from build123d import *

# Parameters (mm, degrees)
BOX001_W          = 17
BOX001_H          = 14.6
BOX001_DEPTH      = 16.5
CYLINDER005_R     = 2.1
CYLINDER005_DEPTH = 2
CYLINDER004_R     = 2.1
CYLINDER004_DEPTH = 2
CYLINDER007_R     = 3.5
CYLINDER007_DEPTH = 0.75
BOX_W             = 7
BOX_H             = 35
BOX_DEPTH         = 0.75
CYLINDER006_R     = 3.5
CYLINDER006_DEPTH = 0.75
CYLINDER001_R     = 4.5
CYLINDER001_DEPTH = 1.5
CYLINDER_R        = 14
CYLINDER_DEPTH    = 19
BOX003_W          = 1
BOX003_H          = 5
BOX003_DEPTH      = 6
BOX002_W          = 1
BOX002_H          = 5
BOX002_DEPTH      = 6
CYLINDER003_R     = 2.5
CYLINDER003_DEPTH = 8.5


with BuildPart() as cube001:
    # Box001 → Box001 (new body)
    with BuildSketch(Plane(origin=(0, -7.3, 2.5), x_dir=(1, 0, 0), z_dir=(0, 0, 1))):
        with Locations((8.5, 7.3)):
            Rectangle(BOX001_W, BOX001_H)
    extrude(amount=BOX001_DEPTH)


with BuildPart() as cylinder005:
    # Cylinder005 → Cylinder005 (new body)
    with BuildSketch(Plane(origin=(0, 17.5, 18), x_dir=(1, 0, 0), z_dir=(0, 0, 1))):
        Circle(CYLINDER005_R)
    extrude(amount=CYLINDER005_DEPTH)


with BuildPart() as cylinder004:
    # Cylinder004 → Cylinder004 (new body)
    with BuildSketch(Plane(origin=(0, -17.5, 18), x_dir=(1, 0, 0), z_dir=(0, 0, 1))):
        Circle(CYLINDER004_R)
    extrude(amount=CYLINDER004_DEPTH)


with BuildPart() as cylinder007:
    # Cylinder007 → Cylinder007 (new body)
    with BuildSketch(Plane(origin=(0, 17.5, 18), x_dir=(1, 0, 0), z_dir=(0, 0, 1))):
        Circle(CYLINDER007_R)
    extrude(amount=CYLINDER007_DEPTH)


with BuildPart() as cube:
    # Box → Box (new body)
    with BuildSketch(Plane(origin=(-3.5, -17.5, 18), x_dir=(1, 0, 0), z_dir=(0, 0, 1))):
        with Locations((3.5, 17.5)):
            Rectangle(BOX_W, BOX_H)
    extrude(amount=BOX_DEPTH)


with BuildPart() as cut001:
    # Cylinder006 → Cylinder006 (new body)
    with BuildSketch(Plane(origin=(0, -17.5, 18), x_dir=(1, 0, 0), z_dir=(0, 0, 1))):
        Circle(CYLINDER006_R)
    extrude(amount=CYLINDER006_DEPTH)

    # Fusion: union Cylinder007, Cube
    add(cylinder007.part)
    add(cube.part)


with BuildPart() as cut001_1:
    # Fusion placement: moved
    add(cut001.part.moved(Location((0, 0, 0.25))))

    # Cut: cut Cylinder004
    add(cylinder004.part, mode=Mode.SUBTRACT)

    # Cut001: cut Cylinder005
    add(cylinder005.part, mode=Mode.SUBTRACT)


with BuildPart() as cylinder001:
    # Cylinder001 → Cylinder001 (new body)
    with BuildSketch(Plane(origin=(-8, 0, 19), x_dir=(1, 0, 0), z_dir=(0, 0, 1))):
        Circle(CYLINDER001_R)
    extrude(amount=CYLINDER001_DEPTH)


with BuildPart() as cylinder:
    # Cylinder → Cylinder (new body)
    with BuildSketch(Plane.XY):
        Circle(CYLINDER_R)
    extrude(amount=CYLINDER_DEPTH)


with BuildPart() as cube003:
    # Box003 → Box003 (new body)
    with BuildSketch(Plane(origin=(-10.5, -2.5, 23), x_dir=(1, 0, 0), z_dir=(0, 0, 1))):
        with Locations((0.5, 2.5)):
            Rectangle(BOX003_W, BOX003_H)
    extrude(amount=BOX003_DEPTH)


with BuildPart() as cube002:
    # Box002 → Box002 (new body)
    with BuildSketch(Plane(origin=(-6.5, -2.5, 23), x_dir=(1, 0, 0), z_dir=(0, 0, 1))):
        with Locations((0.5, 2.5)):
            Rectangle(BOX002_W, BOX002_H)
    extrude(amount=BOX002_DEPTH)


with BuildPart() as motor:
    # Cylinder003 → Cylinder003 (new body)
    with BuildSketch(Plane(origin=(-8, 0, 20.5), x_dir=(1, 0, 0), z_dir=(0, 0, 1))):
        Circle(CYLINDER003_R)
    extrude(amount=CYLINDER003_DEPTH)

    # Cut002: cut Cube002
    add(cube002.part, mode=Mode.SUBTRACT)

    # Cut003: cut Cube003
    add(cube003.part, mode=Mode.SUBTRACT)

    # Fusion001: union Cube001, Cut001, Cylinder001, Cylinder
    add(cube001.part)
    add(cut001_1.part)
    add(cylinder001.part)
    add(cylinder.part)


with BuildPart() as motor_1:
    # Fusion001 placement: moved
    add(motor.part.moved(Location((8, 0, -10))))


solid = motor_1.part
The listing builds one solid part. Answer for the finished solid, in the listing's coordinates (mm). A direction names the side the tool comes from. Round coordinates to 2 decimals unless told otherwise and drop trailing zeros. Loops run counter-clockwise (first coordinate to the right, second up) from the corner with the lowest first, then second, coordinate; pieces in that order, holes last. Notation, with made-up numbers: M 67.5,-16 L 83.5,-16 A17 cw 83.5,9 Z; hole C -18,45.5 d7. An arc over 180 degrees is marked long. Return JSON: item names as keys, results as strings.
Q1. Find section D-D, the plane x = 0. Determine the outline of the cut face in (y, z).
Results list:
{"outline": "M -11.49,-10 L 11.49,-10 L 11.49,9 L 4.5,9 L 4.5,10.5 L 2.5,10.5 L 2.5,19 L -2.5,19 L -2.5,10.5 L -4.5,10.5 L -4.5,9 L -11.49,9 Z"}
Q2. Find section B-B, the plane y = -17. Determine the outline of the cut face in (x, z).
Results list:
{"outline": "M 4.5,8.25 L 5.96,8.25 L 5.96,9 L 4.5,9 Z; M 10.04,8.25 L 11.5,8.25 L 11.5,9 L 10.04,9 Z"}
Q3. Find section C-C, the plane y = 0. Determine the outline of the cut face in (x, z), plus the area to 4 significant figures.
Results list:
{"outline": "M -6,-10 L 22,-10 L 22,-7.5 L 25,-7.5 L 25,9 L 4.5,9 L 4.5,10.5 L 2.5,10.5 L 2.5,13 L 1.5,13 L 1.5,19 L -1.5,19 L -1.5,13 L -2.5,13 L -2.5,10.5 L -4.5,10.5 L -4.5,9 L -6,9 Z", "area": "625.5 mm2"}
Q4. The mould has two halves that part along X. Classify faces 1 (the face through (7.727, -15.418, 8.62)), 2 (the face through (-4.496, 0.198, 9.74)), 3 (the face through (1.5, 0, 16)), 4 (the face through (2, -2, 10.5)): released by +X, released by -X, zero draft, split by the parting line, or undercut.
Results list:
{"face 1": "undercut", "face 2": "split by the parting line", "face 3": "released by +X", "face 4": "zero draft"}
Q5. Which of the six approach directions +Z, -Z, +X, -X, +Y, -Y give full straight-line access (tool end or side, diameter ignored) to faces 5 (the face through (-5.986, 0.616, -0.633)), 6 (the face through (-1.5, 0, 16)), 7 (the face through (22, 7.3, 1)), 8 (the face through (2, 0, 13)), 9 (the face through (1.15, -2.22, 13.75))?
Results list:
{"face 5": "-Z", "face 6": "+Z, -X, +Y, -Y", "face 7": "+Z, -Z, +X, +Y", "face 8": "+Z, +X, +Y, -Y", "face 9": "+Z"}
Q6. Find the intervals of material crossed by line 1 along X through (y, z) = (-17.5, 8.85); line 2 along Y through (x, z) = (8, 8.8); line 3 along Z through (x, y) = (3.5, 1), in increasing order. Write a range as from..to.
Results list:
{"line 1": "x = 4.5..5.9, 10.1..11.5", "line 2": "y = -21..-19.6, -15.4..15.4, 19.6..21", "line 3": "z = -10..10.5"}
Q7. Each of these flat-tipped pins is pushed along its axis until it touches: pin 1 Ø1 at (x, y) = (11, 15) entering from -Z; pin 2 Ø9.5 at (x, y) = (12, 8) entering from +Z; pin 3 Ø0.6 at (y, z) = (15, 8.5) entering from -X; pin 4 Ø1.1 at (x, y) = (-2, 0.5) entering from +Z. Where does it stop, or does it pass through?
Results list:
{"pin 1": "stops at z = 8.25", "pin 2": "stops at z = 9", "pin 3": "stops at x = 4.5", "pin 4": "stops at z = 19"}
Q8. Find section A-A, the plane x = 8. Determine the outline of the cut face in (y, z).
Results list:
{"outline": "M -21,8.25 L -19.6,8.25 L -19.6,9 L -21,9 Z; M -15.4,8.25 L -14,8.25 L -14,-10 L 14,-10 L 14,8.25 L 15.4,8.25 L 15.4,9 L -15.4,9 Z; M 19.6,8.25 L 21,8.25 L 21,9 L 19.6,9 Z"}
